Verification items for this drawing (mm, ordinates from the low corner). Round coordinates to 2 decimals unless told otherwise and drop trailing zeros. Write each loop counter-clockwise with the first axis right and the second up, starting at its lowest first coordinate (ties: lowest second). Pieces come first, ordered by that corner, then holes. Notation, with made-up numbers: (22, 87) -> (27, 87) arc R23 cw to (27, 98) -> close; hole circle Ø4 at (-27.5, 47.25). An arc over 180 degrees is marked (long way). Put each result on its own line as item: value. Start each with the question number.
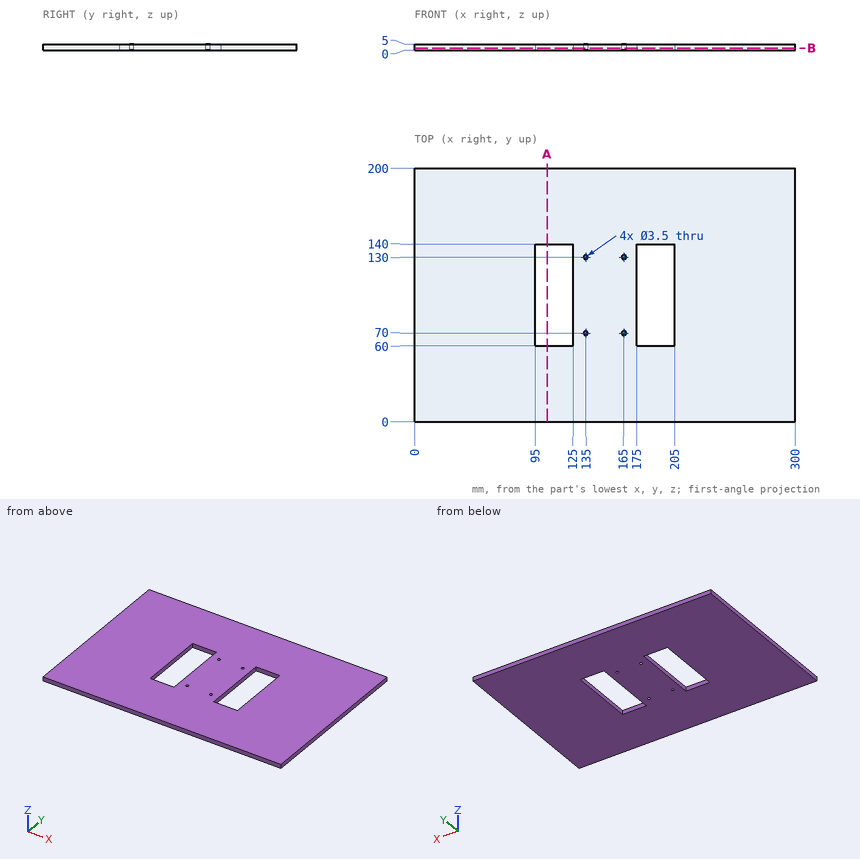
1. Section check B-B, the plane z = 1.8. Enter the section's corners in (x, y).
2. Material ranges on L1, parallel to X at y = 63, z = 1.8; L2, parallel to X at y = 130, z = 1.4; L3, parallel to Y at x = 165, z = 2.6, recorded low to high. Write a range as [from, to].
3. Section check A-A, the plane x = 104.5. Enter the section's corners in (y, z).
Reply:
1. outline: (0, 0) -> (300, 0) -> (300, 200) -> (0, 200) -> close; hole (95, 60) -> (125, 60) -> (125, 140) -> (95, 140) -> close; hole circle Ø3.5 at (135, 70); hole circle Ø3.5 at (135, 130); hole circle Ø3.5 at (165, 70); hole circle Ø3.5 at (165, 130); hole (175, 60) -> (205, 60) -> (205, 140) -> (175, 140) -> close
2. L1: x = [0, 95], [125, 175], [205, 300]
2. L2: x = [0, 95], [125, 133.25], [136.75, 163.25], [166.75, 175], [205, 300]
2. L3: y = [0, 68.25], [71.75, 128.25], [131.75, 200]
3. outline: (0, 0) -> (60, 0) -> (60, 5) -> (0, 5) -> close; (140, 0) -> (200, 0) -> (200, 5) -> (140, 5) -> close
